The model under review builds one solid part; all positions refer to its coordinate system, in mm. Face numbers are marked on the shaded views. A direction names the side the tool comes from. Give positions to 0.01 mm unless a question says otherwise; leave off trailing zeros. Loops run counter-clockwise (first coordinate to the right, second up) from the corner with the lowest first, then second, coordinate; pieces in that order, holes last. Notation, with made-up numbers: M -37.5,24 L -20.5,24 A14 ccw -20.5,42 Z; hole C -36,32 d9. An arc over 180 degrees is marked long. Write item = value, one per line. Start each with the question number.
1. We need section D-D on y = -30. Give the boundary of the cut face in (x, z).
2. We need section A-A on x = -19.05. Give the boundary of the cut face in (y, z), then the cut area to 3 significant figures.
3. For the marked faces 4, 5 and 6, list the 3-axis set-ups (+Z, -Z, +X, -X, +Y, -Y) from which the entire face can be reached by the end or side of a thin tool; tool diameter is ignored.
4. For pin 1 (6.5 mm diameter, centred on x = 19.05, y = 13.081, fed in from -Z), flat-tipped, find the tip position at first contact; note if it passes through.
5. We need section C-C on z = 4. Count the separate pieces of the cut face and the enclosed holes in it, then the cut area to 3 significant figures.
6. We need section B-B on x = 11.5. Give the boundary of the cut face in (y, z) (3 decimals), then the cut area to 3 significant figures.
7. Wall thickness on line 1 along X through (y, z) = (20.5, 5.5); line 2 along X through (y, z) = (0.5, 6); line 3 along Y through (x, z) = (10.16, 11.25): over which ranges is each line inside the solid? List them lowest first. Write a range as from..to.
8. Draft analysis for pull direction X (two halves, no side actions). For the marked faces 1, 2 and 3, state which applies: pulls with the +X half, pulls with the -X half, needs draft (parallel to the pull), parting line crosses it, or undercut.
from build123d import *

# Parameters (mm, degrees)
SKETCH1_W                                       = 50.8
SKETCH1_H                                       = 50.8
SKETCH1_R                                       = 2.5527
SKETCH1_R_2                                     = 7.9375
BOSS_EXTRUDE1_DEPTH                             = 12.7
SKETCH2_W                                       = 50.8
SKETCH2_H                                       = 12.7
BOSS_EXTRUDE2_DEPTH                             = 12.7
CBORE_FOR_10_SOCKET_HEAD_CAP_SCREW1_D           = 5.1054
CBORE_FOR_10_SOCKET_HEAD_CAP_SCREW1_CBORE_D     = 7.9248
CBORE_FOR_10_SOCKET_HEAD_CAP_SCREW1_CBORE_DEPTH = 4.826
SKETCH6_R                                       = 3.9624
CUT_EXTRUDE1_DEPTH                              = 4.826


with BuildPart() as part:
    # Sketch1 → Boss-Extrude1 (new body)
    with BuildSketch(Plane.XY):
        Rectangle(SKETCH1_W, SKETCH1_H)
        with Locations(Location((-19.05, 20.701, 0), (0, 0, 180))):
            Circle(SKETCH1_R, mode=Mode.SUBTRACT)
        with Locations((19.05, 20.701)):
            Circle(SKETCH1_R, mode=Mode.SUBTRACT)
        with Locations((19.05, -17.399)):
            Circle(SKETCH1_R, mode=Mode.SUBTRACT)
        with Locations((10.16, -17.399)):
            Circle(SKETCH1_R, mode=Mode.SUBTRACT)
        with Locations((14.605, 0)):
            Circle(SKETCH1_R_2, mode=Mode.SUBTRACT)
    extrude(amount=BOSS_EXTRUDE1_DEPTH)

    # Sketch2 → Boss-Extrude2 (add)
    with BuildSketch(Plane.XZ.offset(25.4)):
        with Locations((0, 6.35)):
            Rectangle(SKETCH2_W, SKETCH2_H)
    extrude(amount=BOSS_EXTRUDE2_DEPTH)

    # CBORE for #10 Socket Head Cap Screw1 (through all)
    with Locations(Plane(origin=(-24.721209515, -12.864288698, 0), x_dir=(1, 0, 0), z_dir=(0, 0, -1))):
        with Locations((43.771209515, 18.504711302), (43.771209515, -25.945288698)):
            CounterBoreHole(CBORE_FOR_10_SOCKET_HEAD_CAP_SCREW1_D / 2, CBORE_FOR_10_SOCKET_HEAD_CAP_SCREW1_CBORE_D / 2, CBORE_FOR_10_SOCKET_HEAD_CAP_SCREW1_CBORE_DEPTH)

    # Sketch6 → Cut-Extrude1 (cut)
    with BuildSketch(Plane(origin=(0, 0, 12.7), x_dir=(-1, 0, 0), z_dir=(0, 0, -1))):
        with Locations((-19.05, 20.701)):
            Circle(SKETCH6_R)
        with Locations((-19.05, -17.399)):
            Circle(SKETCH6_R)
        with Locations((-10.16, -17.399)):
            Circle(SKETCH6_R)
        with Locations((19.05, 20.701)):
            Circle(SKETCH6_R)
    extrude(amount=CUT_EXTRUDE1_DEPTH, mode=Mode.SUBTRACT)


solid = part.part
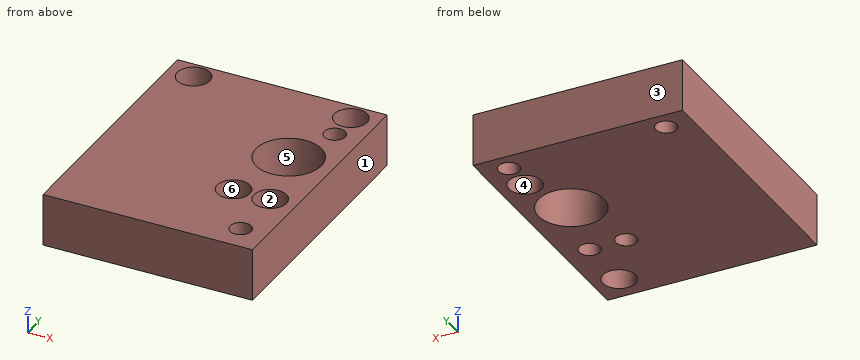
Final values:
q1.outline = M -25.4,0 L 15.33,0 L 15.33,4.83 L 16.9,4.83 L 16.9,12.7 L -25.4,12.7 Z; M 21.2,4.83 L 22.77,4.83 L 22.77,0 L 25.4,0 L 25.4,12.7 L 21.2,12.7 Z
q2.outline = M -38.1,0 L 18.15,0 L 18.15,7.87 L 16.74,7.87 L 16.74,12.7 L -38.1,12.7 Z; M 23.25,0 L 25.4,0 L 25.4,12.7 L 24.66,12.7 L 24.66,7.87 L 23.25,7.87 Z
q2.area = 728 mm²
q3.face_4 = -Z
q3.face_5 = +Z, -Z
q3.face_6 = +Z
q4.pin_1 = 4.83
q5.separate_pieces = 1
q5.enclosed_holes = 7
q5.area = 2,850 mm²
q6.outline = M -38.1,0 L -19.572,0 L -19.572,7.874 L -21.128,7.874 L -21.128,12.7 L -38.1,12.7 Z; M -15.226,0 L -7.305,0 L -7.305,12.7 L -13.67,12.7 L -13.67,7.874 L -15.226,7.874 Z; M 7.305,0 L 25.4,0 L 25.4,12.7 L 7.305,12.7 Z
q6.area = 551 mm²
q7.line_1 = -25.4..-21.59, -16.51..16.51, 21.59..25.4
q7.line_2 = -25.4..6.68, 22.53..25.4
q7.line_3 = -38.1..-21.36, -13.44..-6.58, 6.58..25.4
q8.face_1 = pulls with the +X half
q8.face_2 = undercut
q8.face_3 = needs draft
